Part print with two shaded views. Sizes in mm from the minimum x, y, z corner. Give positions to 0.01 mm unless a question says otherwise; leave off trailing zeros. Write each loop counter-clockwise with the first axis right and the second up, starting at its lowest first coordinate (ties: lowest second). Pieces come first, ordered by that corner, then holes. Notation, with made-up numbers: (47, 75) -> (88, 75) arc R14 ccw to (88, 100) -> close; hole circle Ø10 at (2.5, 69). An arc over 180 degrees is marked (long way). Write item = value, one per line. Start each with the question number.
Q1. Drop flat-ended pins along their axis: P1, Ø1.5, axis at x = 17, z = 7.5, coming from the +Y side (1 decimal); P2, Ø1, axis at x = 14, z = 2.5, coming from the -Y side; P3, Ø5, axis at x = 3.5, y = 5, coming from the -Z side; P4, Ø1.9, axis at y = 18, z = 6, coming from the +X side (1 decimal). Give the stop position or say it passes through.
Q2. Wall check: line 1 (X direction, y = 11, z = 5.75) (1 decimal); line 2 (Y direction, x = 11.75, z = 2.75); line 3 (X direction, y = 13.5, z = 2.25) (1 decimal). Give the ranges that are in metal, low to high.
Q3. Saw through at A-A, the plane z = 1.75. List the corners of the cut face in (x, y) (1 decimal).
Q4. Mould opens along X. For the marked faces 1, 2 and 3 say: pulls with the +X half, pulls with the -X half, needs draft (parallel to the pull), parting line crosses it, or undercut.
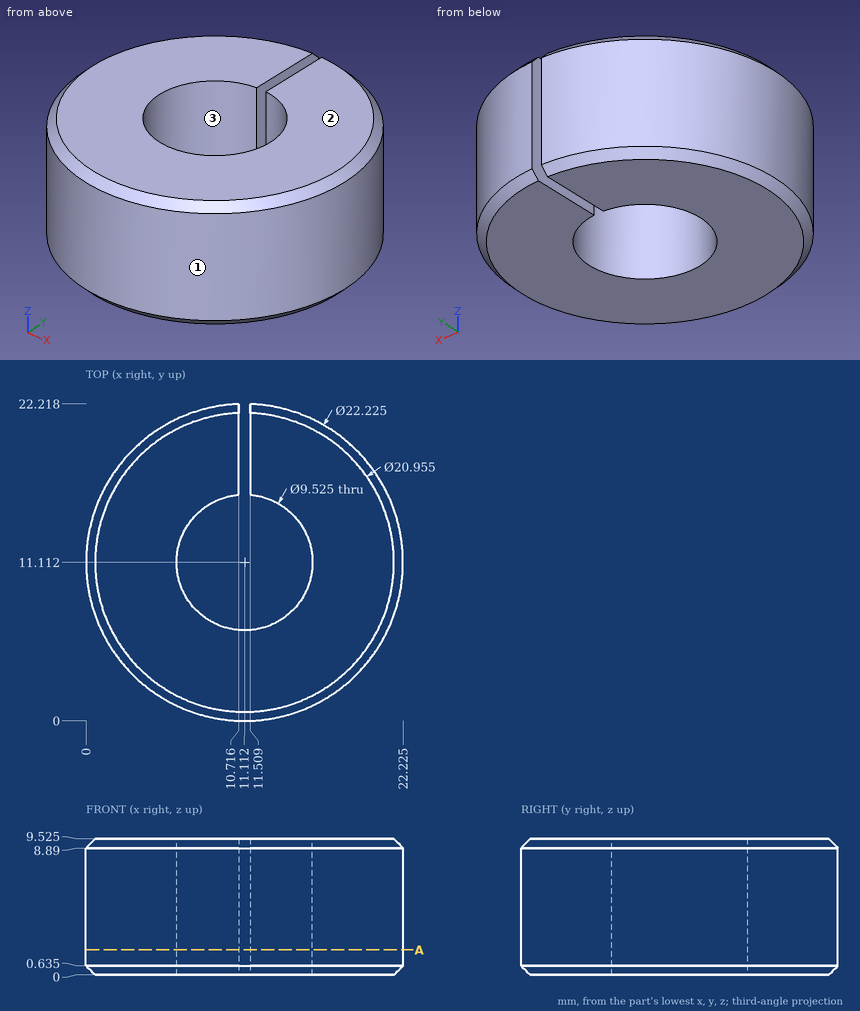
Report:
q1.P1 = 21
q1.P2 = 0.26
q1.P3 = 0
q1.P4 = 20.5
q2.line_1 = 0 to 6.4, 15.9 to 22.2
q2.line_2 = 0.02 to 6.39, 15.83 to 22.21
q2.line_3 = 0.3 to 7, 15.2 to 22
q3.outline = (10.7, 15.9) -> (10.7, 22.2) arc R11.1 ccw (long way) to (11.5, 22.2) -> (11.5, 15.9) arc R4.8 cw (long way) to start
q4.face_1 = parting line crosses it
q4.face_2 = needs draft
q4.face_3 = undercut
